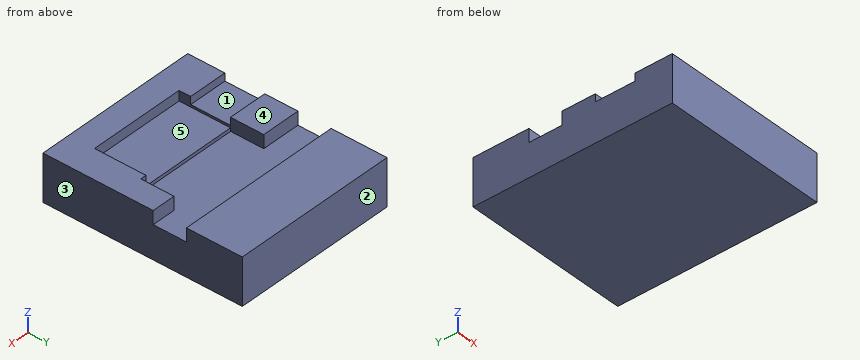
```python
from build123d import *

# Parameters (mm, degrees)
F0_W     = 50
F0_H     = 60
F1_DEPTH = 14
F2_W     = 29.2
F2_H     = 15.5
F3_DEPTH = 3
F4_W     = 11.810996
F4_H     = 12
F5_DEPTH = 2.3
F7_DEPTH = 4


with BuildPart() as f1:
    # F0 (on Top) → F1 (new body)
    with BuildSketch(Plane.XY):
        with Locations((-0.093784, -7.974683)):
            Rectangle(F0_W, F0_H)
    extrude(amount=F1_DEPTH)

    # F2 (on face) → F3 (cut)
    with BuildSketch(Plane.XY.offset(14)):
        with Locations((1.317212, -22.539393)):
            Rectangle(F2_W, F2_H)
    extrude(amount=-F3_DEPTH, mode=Mode.SUBTRACT)

    # F4 (on face) → F5 (cut)
    with BuildSketch(Plane.XY.offset(14)):
        with Locations((-19.188286, -20.789393)):
            Rectangle(F4_W, F4_H)
    extrude(amount=-F5_DEPTH, mode=Mode.SUBTRACT)

    # F6 (on face) → F7 (cut)
    with BuildSketch(Plane.XY.offset(14)):
        Polygon((-13.282784, -4.789393), (-13.282784, -14.789393), (15.917212, -14.789393), (17.717216, -14.789393), (17.717216, -4.789393), (24.906216, -4.789393), (24.906216, 5.210607), (17.717216, 5.210607), (-13.282784, 5.210607), (-25.093784, 5.210607), (-25.093784, -4.789393), align=None)
    extrude(amount=-F7_DEPTH, mode=Mode.SUBTRACT)


solid = f1.part
```
Could you check a few things on this model? Use its own coordinates, in mm. Face numbers are marked on the shaded views. A direction names the side the tool comes from. Coordinates: 2 decimals unless noted, no trailing zeros. Order: outer loops, then holes, each group sorted by start corner. A loop starts at its lowest first (then second) coordinate and runs counter-clockwise, first axis right, second up. Notation, with made-up numbers: M 59,-14 L 75,-14 A27 ccw 75,23 Z; hole C 10,-20.5 d2. An arc over 180 degrees is marked long. Use a Markdown table: item, result. Add a question column.
Q1. I want a section at C-C on x = -21. List the corners of the cut face in (y, z) for me.
Q2. I want a section at A-A on y = -25. List the corners of the cut face in (x, z) for me, then the cut area to 3 significant figures.
Q3. If I drill on L1, parallel to Y at x = -13.5, z = 13.25; L2, parallel to Y at x = 17.5, z = 12.25; L3, parallel to Z at x = 11.5, y = -1, over which ranges is the centre line in solid material (lowest first)?
Q4. We'd pull the mould along Y, two halves only. Please class the marked faces 1, 2 and 3: pulls with the +Y half, pulls with the -Y half, needs draft (parallel to the pull), parting line crosses it, or undercut.
Q5. I want a section at B-B on x = -1. List the corners of the cut face in (y, z) for me, then the cut area to 4 significant figures.
Q6. I'm going to push flat-ended pins straight in: pin 1 (6 mm diameter, centred on x = -17.5, y = -18.5, fed in from +Z); pin 2 (0.9 mm diameter, centred on y = -25, z = 13, fed in from -X); pin 3 (6 mm diameter, centred on x = 7.5, y = -6, fed in from +Z). Where does each tip first touch, or does it pass through?
Q7. Which directions (+Z, -Z, +X, -X, +Y, -Y) give clear straight access to the entire face, cutting with the end or side of a thin tool? Please do the marked faces 4 and 5.
Checked values:
| question | item | result |
|---|---|---|
| 1 | outline | M -37.97,0 L 22.03,0 L 22.03,14 L 5.21,14 L 5.21,10 L -4.79,10 L -4.79,14 L -14.79,14 L -14.79,11.7 L -26.79,11.7 L -26.79,14 L -37.97,14 Z |
| 2 | outline | M -25.09,0 L 24.91,0 L 24.91,14 L 15.92,14 L 15.92,11 L -13.28,11 L -13.28,11.7 L -25.09,11.7 Z |
| 2 | area | 585 mm² |
| 3 | L1 | -37.97 to -26.79, -14.79 to -4.79, 5.21 to 22.03 |
| 3 | L2 | -37.97 to -14.79, 5.21 to 22.03 |
| 3 | L3 | 0 to 10 |
| 4 | face 1 | undercut |
| 4 | face 2 | pulls with the +Y half |
| 4 | face 3 | needs draft |
| 5 | outline | M -37.97,0 L 22.03,0 L 22.03,14 L 5.21,14 L 5.21,10 L -14.79,10 L -14.79,11 L -30.29,11 L -30.29,14 L -37.97,14 Z |
| 5 | area | 713.5 mm² |
| 6 | pin 1 | z = 11.7 |
| 6 | pin 2 | x = 15.92 |
| 6 | pin 3 | z = 10 |
| 7 | face 4 | +Z, +X, -X, +Y, -Y |
| 7 | face 5 | +Z |
